```python
from build123d import *

# Parameters (mm, degrees)
SKETCH1_W            = 150
SKETCH1_H            = 180
BOSS_EXTRUDE1_DEPTH  = 110
SKETCH2_W            = 35
SKETCH2_H            = 10
CUT_EXTRUDE1_DEPTH   = 228
BOSS_EXTRUDE2_DEPTH  = 40
SKETCH5_R            = 40
SKETCH5_R_2          = 5
BOSS_EXTRUDE3_DEPTH  = 40
BOSS_EXTRUDE5_DEPTH  = 40
CUT_EXTRUDE2_DEPTH   = 40
BOSS_EXTRUDE6_DEPTH  = 40
CUT_EXTRUDE3_START   = -40
CUT_EXTRUDE3_DEPTH   = 40
BOSS_EXTRUDE7_START  = -30
SKETCH11_R           = 5
BOSS_EXTRUDE7_DEPTH  = 30
SKETCH12_R           = 5
BOSS_EXTRUDE8_DEPTH  = 30
CUT_EXTRUDE4_DEPTH   = 187
BOSS_EXTRUDE9_START  = 90
SKETCH16_R           = 5
BOSS_EXTRUDE9_DEPTH  = 90
BOSS_EXTRUDE10_START = 3.5
SKETCH17_R           = 7.5
SKETCH17_R_2         = 5
BOSS_EXTRUDE10_DEPTH = 3.5
SKETCH18_R           = 7.5
SKETCH18_R_2         = 5
BOSS_EXTRUDE11_DEPTH = 3.5
SKETCH20_R           = 11.405
CUT_EXTRUDE5_DEPTH   = 20


with BuildPart() as part:
    # Sketch1 → Boss-Extrude1 (new body)
    with BuildSketch(Plane.XY):
        Rectangle(SKETCH1_W, SKETCH1_H)
    extrude(amount=BOSS_EXTRUDE1_DEPTH)

    # Sketch2 → Cut-Extrude1 (cut)
    with BuildSketch(Plane(origin=(0, 90, 0), x_dir=(1, 0, 0), z_dir=(0, 1, 0))):
        with Locations((17.5, -5)):
            Rectangle(SKETCH2_W, SKETCH2_H)
        with Locations((-17.5, -5)):
            Rectangle(SKETCH2_W, SKETCH2_H)
    extrude(amount=-CUT_EXTRUDE1_DEPTH, mode=Mode.SUBTRACT)

    # Sketch3 → Boss-Extrude2 (add)
    with BuildSketch(Plane(origin=(-35, 0, 0), x_dir=(0, 0, -1), z_dir=(1, 0, 0))):
        with BuildLine():
            Line((50, 90), (0, 90))
            Line((0, 90), (0, 50))
            Line((0, 50), (10, 50))
            ThreePointArc((10, 50), (21.715728753, 78.284271247), (50, 90))
        make_face()
        with BuildLine():
            Line((10, 50), (0, 50))
            Line((0, 50), (0, -85.77))
            Line((0, -85.77), (2.99, -85.77))
            Line((2.99, -85.77), (82.660422477, 26.906780138))
            ThreePointArc((82.660422477, 26.906780138), (37.884243711, 11.879028743), (10, 50))
        make_face()
        with BuildLine():
            ThreePointArc((90, 50), (78.284271247, 78.284271247), (50, 90))
            Line((50, 90), (50, 55))
            ThreePointArc((50, 55), (53.535533906, 53.535533906), (55, 50))
            ThreePointArc((55, 50), (50, 45), (45, 50))
            Line((45, 50), (10, 50))
            ThreePointArc((10, 50), (37.884243711, 11.879028743), (82.660422477, 26.906780138))
            ThreePointArc((82.660422477, 26.906780138), (88.120971257, 37.884243711), (90, 50))
        make_face()
        with BuildLine():
            Line((50, 55), (50, 90))
            ThreePointArc((50, 90), (21.715728753, 78.284271247), (10, 50))
            Line((10, 50), (45, 50))
            ThreePointArc((45, 50), (46.464466094, 53.535533906), (50, 55))
        make_face()
    extrude(amount=-BOSS_EXTRUDE2_DEPTH)

    # Sketch5 → Boss-Extrude3 (add)
    # profile 1 of 2: a face of its own
    with BuildSketch(Plane(origin=(75, 0, 0), x_dir=(0, 0, -1), z_dir=(1, 0, 0))):
        with BuildLine():
            Line((50, 90), (0, 90))
            Line((0, 90), (0, -85.77))
            Line((0, -85.77), (2.99, -85.77))
            Line((2.99, -85.77), (82.660422477, 26.906780138))
            ThreePointArc((82.660422477, 26.906780138), (14.477269288, 31.61153615), (50, 90))
        make_face()
    # profile 2 of 2: a face of its own
    with BuildSketch(Plane(origin=(75, 0, 0), x_dir=(0, 0, -1), z_dir=(1, 0, 0))):
        with Locations((50, 50)):
            Circle(SKETCH5_R)
        with Locations((50, 50)):
            Circle(SKETCH5_R_2, mode=Mode.SUBTRACT)
    extrude(amount=-BOSS_EXTRUDE3_DEPTH)

    # Sketch6 → Boss-Extrude5 (add)
    with BuildSketch(Plane(origin=(75, 0, 0), x_dir=(0, 0, -1), z_dir=(1, 0, 0))):
        Polygon((2.99, -85.77), (0, -90), (0, -85.77), align=None)
    extrude(amount=-BOSS_EXTRUDE5_DEPTH)

    # Sketch8 → Cut-Extrude2 (cut)
    with BuildSketch(Plane.ZY.offset(-35)):
        with BuildLine():
            Line((0, -90), (5.18, -90))
            ThreePointArc((5.18, -90), (0.670947119, -88.704033579), (-2.99, -85.77))
            Line((-2.99, -85.77), (0, -90))
        make_face()
    extrude(amount=-CUT_EXTRUDE2_DEPTH, mode=Mode.SUBTRACT)

    # Sketch9 → Boss-Extrude6 (add)
    with BuildSketch(Plane.ZY.offset(75)):
        Polygon((-2.99, -85.77), (0, -90), (0, -85.77), align=None)
    extrude(amount=-BOSS_EXTRUDE6_DEPTH)

    # Sketch10 → Cut-Extrude3 (cut)
    with BuildSketch(Plane(origin=(-35, 0, 0), x_dir=(0, 0, -1), z_dir=(1, 0, 0)).offset(CUT_EXTRUDE3_START)):
        with BuildLine():
            Line((-5.18, -90), (0, -90))
            Line((0, -90), (2.99, -85.77))
            ThreePointArc((2.99, -85.77), (-0.670947119, -88.704033579), (-5.18, -90))
        make_face()
    extrude(amount=CUT_EXTRUDE3_DEPTH, mode=Mode.SUBTRACT)

    # Sketch11 → Boss-Extrude7 (add)
    with BuildSketch(Plane.ZY.offset(75).offset(BOSS_EXTRUDE7_START)):
        with Locations(Location((-50, 50, 0), (0, 0, 180))):
            Circle(SKETCH11_R)
    extrude(amount=BOSS_EXTRUDE7_DEPTH)

    # Sketch12 → Boss-Extrude8 (add)
    with BuildSketch(Plane(origin=(75, 0, 0), x_dir=(0, 0, -1), z_dir=(1, 0, 0))):
        with Locations((50, 50)):
            Circle(SKETCH12_R)
    extrude(amount=-BOSS_EXTRUDE8_DEPTH)

    # Sketch14 → Cut-Extrude4 (cut)
    with BuildSketch(Plane(origin=(0, 90, 0), x_dir=(1, 0, 0), z_dir=(0, 1, 0))):
        Polygon((-60, 50), (-50, 90), (-75, 90), (-75, 50), align=None)
        Polygon((-75, -10), (-60, 50), (-75, 50), (-75, 0), align=None)
        Polygon((60, 50), (75, -10), (75, 0), (75, 50), align=None)
        Polygon((50, 90), (60, 50), (75, 50), (75, 90), align=None)
    extrude(amount=-CUT_EXTRUDE4_DEPTH, mode=Mode.SUBTRACT)

    # Sketch16 → Boss-Extrude9 (add)
    with BuildSketch(Plane(origin=(-45, 0, 0), x_dir=(0, 0, -1), z_dir=(1, 0, 0)).offset(BOSS_EXTRUDE9_START)):
        with Locations((50, 50)):
            Circle(SKETCH16_R)
    extrude(amount=-BOSS_EXTRUDE9_DEPTH)

    # Sketch17 → Boss-Extrude10 (add)
    with BuildSketch(Plane(origin=(-35, 0, 0), x_dir=(0, 0, -1), z_dir=(1, 0, 0)).offset(BOSS_EXTRUDE10_START)):
        with Locations((50, 50)):
            Circle(SKETCH17_R)
        with Locations((50, 50)):
            Circle(SKETCH17_R_2, mode=Mode.SUBTRACT)
    extrude(amount=-BOSS_EXTRUDE10_DEPTH)

    # Sketch18 → Boss-Extrude11 (add)
    with BuildSketch(Plane.ZY.offset(-35)):
        with Locations(Location((-50, 50, 0), (0, 0, 180))):
            Circle(SKETCH18_R)
        with Locations((-50, 50)):
            Circle(SKETCH18_R_2, mode=Mode.SUBTRACT)
    extrude(amount=BOSS_EXTRUDE11_DEPTH)

    # Sketch20 → Cut-Extrude5 (cut)
    with BuildSketch(Plane.XY.offset(110)):
        with Locations((0, 50)):
            Circle(SKETCH20_R)
    extrude(amount=-CUT_EXTRUDE5_DEPTH, mode=Mode.SUBTRACT)


solid = part.part
```
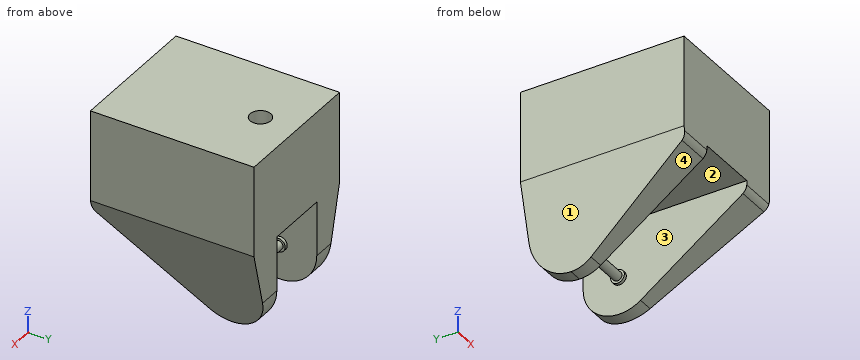
The listing builds one solid part. Answer for the finished solid, in the listing's coordinates (mm). Face numbers are marked on the shaded views. Coordinates: 2 decimals unless noted, no trailing zeros. Write each loop counter-clockwise with the first axis right and the second up, starting at its lowest first coordinate (ties: lowest second). Pieces come first, ordered by that corner, then holes. Notation, with made-up numbers: (31, -27) - (67, -27) arc R24 ccw to (67, 8) - close; hole circle Ø6 at (62, 51). An arc over 180 degrees is marked (long way). Return JSON: item names as keys, results as strings. Group by question number.
Q1. The part is cut by section A-A on x = 21. Write down the section's boundary in (y, z), and give its area (3 significant figures).
Q2. The part is cut by section B-B on z = -21. Write down the section's boundary in (x, y), and give its area (3 significant figures).
Q3. Flat-ended cylindrical pins translate along their axes: pin 1 Ø3 at (x, z) = (-38.5, -9.5) entering from -Y; pin 2 Ø12 at (x, z) = (-50, -52) entering from +Y; pin 3 Ø1.5 at (y, z) = (6, -19.5) entering from -X; pin 4 Ø4.5 at (y, z) = (47, -48.5) entering from -X. Find the tip coordinate at first contact, or state that the pin passes through.
Q4. For a pull along X with two mould halves and no side action, classify the marked faces 1, 2, 3 and 4 as +X half, -X half, draft (parallel to the pull), parting line (faces both ways), or undercut.
Q5. The part is cut by section C-C on y = 69. Write down the section's boundary in (x, z).
Q6. Find the intervals of material crossed by line 1 along Y through (x, z) = (0, 94) (3 decimals); line 2 along X through (y, z) = (-75.5, -9.5) (3 decimals); line 3 along X through (y, z) = (34, 5.5) (3 decimals), in increasing order. Write a range as [from, to].
Q7. The part is cut by section D-D on x = 0. Write down the section's boundary in (y, z) (3 decimals), and give its area (3 significant figures).
Evaluation:
{
 "1": {"outline": "(-90, 10) - (90, 10) - (90, 110) - (-90, 110) - close; circle Ø10 at (50, -50)", "area": "18,100 mm2"},
 "2": {"outline": "(-67.25, -60.3) - (-35, -60.3) - (-35, 90) - (-67.25, 90) - close; (35, -60.3) - (67.25, -60.3) - (67.25, 90) - (35, 90) - close", "area": "9,690 mm2"},
 "3": {"pin 1": "stops at y = -78.68", "pin 2": "stops at y = 90", "pin 3": "stops at x = -67.81", "pin 4": "stops at x = -60.94"},
 "4": {"face 1": "-X half", "face 2": "undercut", "face 3": "undercut", "face 4": "draft"},
 "5": {"outline": "(-75, 10) - (-51.2, -85.2) - (-35, -85.2) - (-35, 10) - (35, 10) - (35, -85.2) - (51.2, -85.2) - (75, 10) - (75, 110) - (-75, 110) - close"},
 "6": {"line 1": "y = [-90, 38.595], [61.405, 90]", "line 2": "x = [-70.125, -35], [35, 70.125]", "line 3": "x = [-73.875, -35], [35, 73.875]"},
 "7": {"outline": "(-90, 10) - (90, 10) - (90, 110) - (61.405, 110) - (61.405, 90) - (38.595, 90) - (38.595, 110) - (-90, 110) - close; circle Ø10 at (50, -50)", "area": "17,600 mm2"}
}
